For this review, use the dimensioned drawing (mm, ordinates from the lowest corner) and the shaded views. Give positions to 0.01 mm unless a question says otherwise; leave off trailing zeros. Loops run counter-clockwise (first coordinate to the right, second up) from the corner with the lowest first, then second, coordinate; pieces in that order, holes last. Notation, with made-up numbers: M 7.5,-39 L 29.5,-39 A18 ccw 29.5,-6 Z; hole C -11,20.25 d10. An arc over 180 degrees is marked long. Return JSON: item names as keys, results as strings.
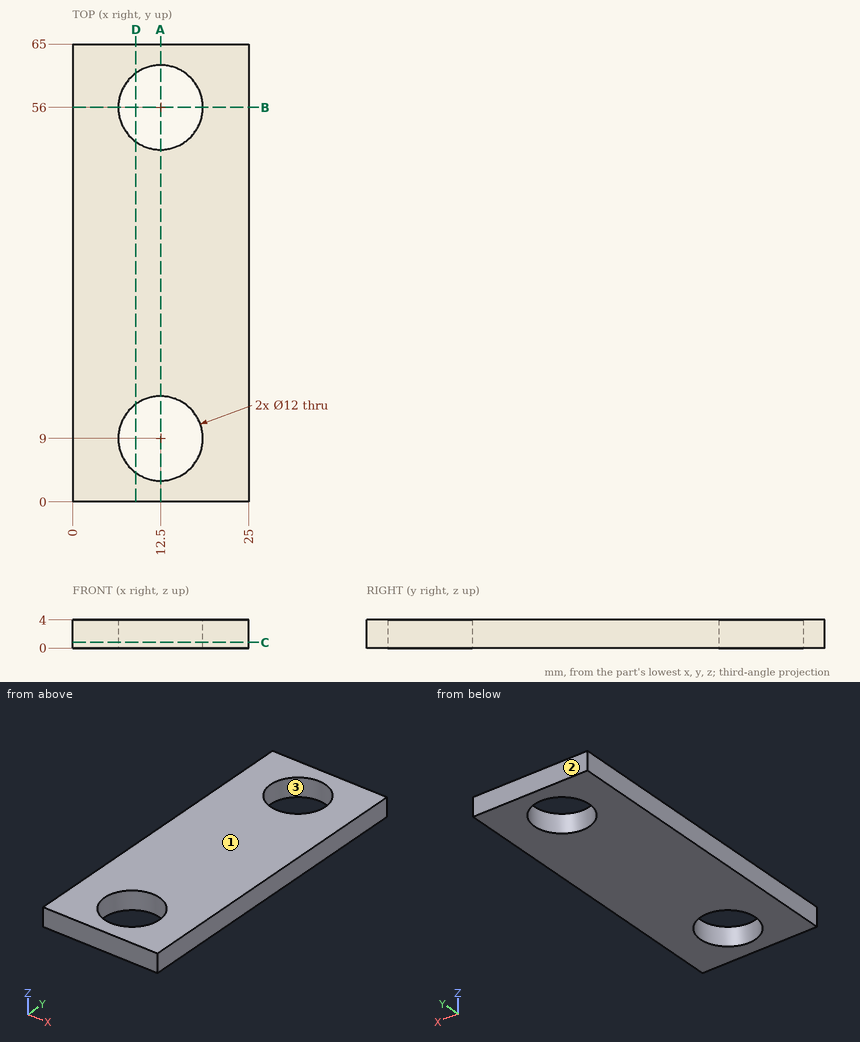
1) The part is to be moulded in two halves that separate along Y. For the marked faces 1, 2 and 3, say which applies: released by +Y, released by -Y, zero draft, split by the parting line, or undercut.
From the geometry:
{"face 1": "zero draft", "face 2": "released by +Y", "face 3": "undercut"}
2) Consider section D-D on x = 9. Write out the cut boundary in (y, z).
From the geometry:
{"outline": "M 0,0 L 4.13,0 L 4.13,4 L 0,4 Z; M 13.87,0 L 51.13,0 L 51.13,4 L 13.87,4 Z; M 60.87,0 L 65,0 L 65,4 L 60.87,4 Z"}
3) Consider section B-B on y = 56. Write out the cut boundary in (x, z).
From the geometry:
{"outline": "M 0,0 L 6.5,0 L 6.5,4 L 0,4 Z; M 18.5,0 L 25,0 L 25,4 L 18.5,4 Z"}
4) Wall thickness on L1, parallel to Y at x = 12.5, z = 1.95; L2, parallel to Y at x = 14.5, z = 2.1; L3, parallel to X at y = 10, z = 2.1: over which ranges is each line inside the solid? List them lowest first. Write a range as from..to.
From the geometry:
{"L1": "0..3, 15..50, 62..65", "L2": "0..3.34, 14.66..50.34, 61.66..65", "L3": "0..6.58, 18.42..25"}
5) Consider section C-C on z = 0.8. Write out the cut boundary in (x, y), then the cut area to 3 significant figures.
From the geometry:
{"outline": "M 0,0 L 25,0 L 25,65 L 0,65 Z; hole C 12.5,9 d12; hole C 12.5,56 d12", "area": "1,400 mm²"}
6) Consider section A-A on x = 12.5. Write out the cut boundary in (y, z).
From the geometry:
{"outline": "M 0,0 L 3,0 L 3,4 L 0,4 Z; M 15,0 L 50,0 L 50,4 L 15,4 Z; M 62,0 L 65,0 L 65,4 L 62,4 Z"}
